CAD build for the part. Positions are in the model's coordinates, mm. Face numbers are marked on the shaded views. A direction names the side the tool comes from. Give positions to 0.01 mm unless a question says otherwise; leave off trailing zeros. Order: outer loops, then holes, each group sorted by start corner. A loop starts at its lowest first (then second) coordinate and runs counter-clockwise, first axis right, second up.
Item 1: Band-saw the part on A-A on y = 0. Give the cut face in (x, z) (3 decimals).
Item 2: Band-saw the part on C-C on x = 12. Give the cut face in (y, z) (3 decimals).
Item 3: Band-saw the part on B-B on z = 0. Give the cut face in (x, y) (3 decimals).
Item 4: Band-saw the part on D-D on z = -33.5. Give the cut face in (x, y).
Item 5: Which spindle directions (+Z, -Z, +X, -X, +Y, -Y) get a long thin tool onto all of the face, cutting with end or side? Do the marked faces 5, 6 and 7. Say none if no direction does.
Item 6: Wall check: L1, parallel to Z at x = 1.9, y = 0 (3 decimals); L2, parallel to Y at x = 2, z = -30; L3, parallel to Y at x = 3.5, z = -47.5. Give the ranges that are in metal, low to high.
Item 7: Flat gauge pins, fed straight in: P1, Ø2, axis at x = 24, y = -3.5, coming from the -Z side; P2, Ø5, axis at x = 7, y = 5, coming from the +Z side; P3, Ø1.5, axis at x = 3.5, z = -17.5, coming from the -Y side. Where does each tip first touch, or does it go through?
Item 8: Two-plate mould, pull along Y, no slides. Class the marked faces 1, 2, 3 and 4: released by +Y, released by -Y, zero draft, split by the parting line, or undercut.
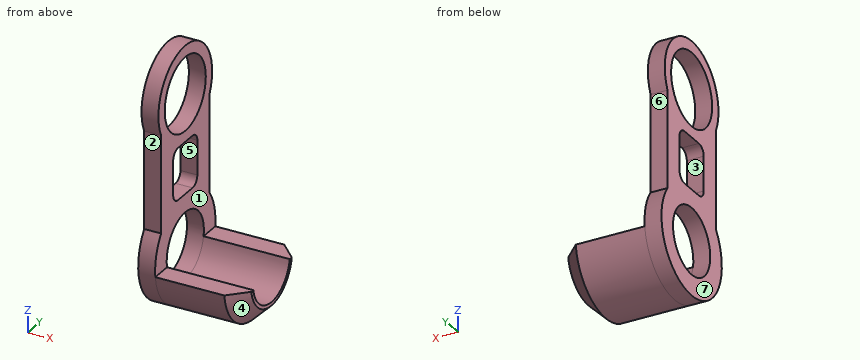
```python
from build123d import *

# Parameters (mm, degrees)
F0_R     = 9.779
F0_W     = 12.7
F0_H     = 15.24
F0_R_2   = 10.795
F1_DEPTH = 4.9800002
F3_DEPTH = 25.4
F4_SIZE  = 5.08
F5_R     = 2.54


# Not quite as in the source:
# - a feature names something its author has since deleted; it is built from what else it names


with BuildPart() as f1:
    # F0 (on Right) → F1 (new body)
    with BuildSketch(Plane.YZ):
        with BuildLine():
            Line((12.7, -34.7691013034), (12.7, -6.1941013034))
            ThreePointArc((12.7, -6.1941013034), (0, 14.12999968), (-12.7, -6.1941013034))
            Line((-12.7, -6.1941013034), (-12.7, -34.7691013034))
            ThreePointArc((-12.7, -34.7691013034), (0, -60.1691013034), (12.7, -34.7691013034))
        make_face()
        with Locations((0, -44.2941013034)):
            Circle(F0_R, mode=Mode.SUBTRACT)
        with Locations((0, -21.59)):
            Rectangle(F0_W, F0_H, mode=Mode.SUBTRACT)
        Circle(F0_R_2, mode=Mode.SUBTRACT)
    extrude(amount=F1_DEPTH)

    # F2 (on face) → F3 (join)
    with BuildSketch(Plane.YZ.offset(4.9800002)):
        with BuildLine():
            ThreePointArc((9.6160052517, -46.0721013034), (0, -54.0731013034), (-9.6160052517, -46.0721013034))
            Line((-9.6160052517, -46.0721013034), (-15.7751177809, -46.0721013034))
            ThreePointArc((-15.7751177809, -46.0721013034), (0, -60.1691013034), (15.7751177809, -46.0721013034))
            Line((15.7751177809, -46.0721013034), (9.6160052517, -46.0721013034))
        make_face()
    extrude(amount=F3_DEPTH)

    # F4
    f4_edges = [f1.edges().sort_by_distance(p)[0] for p in [
        (30.38, 0, -60.169101),
    ]]
    chamfer(f4_edges, length=F4_SIZE)

    # F5
    f5_edges = [f1.edges().sort_by_distance(p)[0] for p in [
        (2.49, 6.35, -13.97),
        (2.49, -6.35, -13.97),
        (2.49, 6.35, -29.21),
        (2.49, -6.35, -29.21),
    ]]
    fillet(f5_edges, radius=F5_R)


solid = f1.part
```
The answers:
1. outline: (0, -60.169) - (25.3, -60.169) - (30.38, -55.089) - (30.38, -54.073) - (0, -54.073) - close; (0, -34.515) - (4.98, -34.515) - (4.98, -29.21) - (0, -29.21) - close; (0, -13.97) - (4.98, -13.97) - (4.98, -10.795) - (0, -10.795) - close; (0, 10.795) - (4.98, 10.795) - (4.98, 14.13) - (0, 14.13) - close
2. outline: (-15.775, -46.072) arc R15.875 ccw to (15.775, -46.072) - (9.616, -46.072) arc R9.779 cw to (-9.616, -46.072) - close
3. outline: (0, -14.13) - (4.98, -14.13) - (4.98, -10.795) - (0, -10.795) - close; (0, 10.795) - (4.98, 10.795) - (4.98, 14.13) - (0, 14.13) - close
4. outline: (0, -12.7) - (4.98, -12.7) - (4.98, 12.7) - (0, 12.7) - close
5. face 5: +X, -X
5. face 6: +X, -X, +Y
5. face 7: +Z, -Z, -X, +Y, -Y
6. L1: z = -60.169 to -54.073, -34.515 to -29.21, -13.97 to -10.795, 10.795 to 14.13
6. L2: y = -12.7 to 12.7
6. L3: y = -15.55 to -9.24, 9.24 to 15.55
7. P1: stops at z = -59.97
7. P2: stops at z = 13.68
7. P3: stops at y = -12.7
8. face 1: zero draft
8. face 2: released by -Y
8. face 3: undercut
8. face 4: split by the parting line
